Check sheet for the modelled part. Datum: model origin and axes. Units: mm. Coordinates: 2 decimals unless noted, no trailing zeros. Write each loop counter-clockwise with the first axis right and the second up, starting at its lowest first coordinate (ties: lowest second). Pieces come first, ordered by that corner, then holes. Notation, with made-up numbers: (-12.5, 61) -> (1.5, 61) arc R18 ccw to (1.5, 90) -> close; hole circle Ø5 at (-35.75, -21.5). An arc over 180 degrees is marked (long way). One line per item, written item: value. Start each with the question number.
1) Sectioned sample at C-C on x = -44.15. Enter the section's corners in (y, z), plus the area to 3 significant figures.
2) Sectioned sample at B-B on y = 3.75. Enter the section's corners in (x, z), plus the area to 3 significant figures.
3) Draft check along Z on faces 1 (the cylindrical face through (-6.5, 6.3, 0.1)), 2 (the flat face through (-29, 12.7, 0)), 3 (the flat face through (-28, 6, -25)), 4 (the flat face through (-29, 6, 25)). Enter one of: +Z half, -Z half, draft (parallel to the pull), parting line (faces both ways), or undercut.
4) Scan lines: line 1 along X through (y, z) = (8.25, 18.5); line 2 along Z through (x, y) = (-3.5, 2); line 3 along X through (y, z) = (5.75, 17). Record each from-to range of solid material in increasing order. Write a range as [from, to].
5) Gauge pin test, flat end, axial feed: P1, Ø3.5, axis at x = -44.15, z = 18.5, coming from the +Y side. Record the tip position at first contact, or that the pin passes through.
6) Sectioned sample at A-A on z = -18.5. Enter the section's corners in (x, y).
7) Sectioned sample at D-D on z = 0. Enter the section's corners in (x, y).
```python
from build123d import *

# Parameters (mm, degrees)
CROQUIS2_R              = 3
SALIENTE_EXTRUIR1_DEPTH = 12.7


with BuildPart() as part:
    # Croquis2 → Saliente-Extruir1 (new body)
    with BuildSketch(Plane(origin=(0, 0, 0), x_dir=(1, 0, 0), z_dir=(0, 1, 0))):
        with BuildLine():
            Line((0, 25), (-57.15, 25))
            Line((-57.15, 25), (-57.15, -25))
            Line((-57.15, -25), (0, -25))
            Line((0, -25), (0, -6.5))
            ThreePointArc((0, -6.5), (-6.5, 0), (0, 6.5))
            Line((0, 6.5), (0, 25))
        make_face()
        with Locations(Location((-44.15, -18.5, 0), (0, 0, 270))):
            Circle(CROQUIS2_R, mode=Mode.SUBTRACT)
        with Locations(Location((-44.15, 18.5, 0), (0, 0, 270))):
            Circle(CROQUIS2_R, mode=Mode.SUBTRACT)
    extrude(amount=SALIENTE_EXTRUIR1_DEPTH)


solid = part.part
```
Answers:
1. outline: (0, -25) -> (12.7, -25) -> (12.7, -21.5) -> (0, -21.5) -> close; (0, -15.5) -> (12.7, -15.5) -> (12.7, 15.5) -> (0, 15.5) -> close; (0, 21.5) -> (12.7, 21.5) -> (12.7, 25) -> (0, 25) -> close
1. area: 483 mm2
2. outline: (-57.15, -25) -> (0, -25) -> (0, -6.5) arc R6.5 cw to (0, 6.5) -> (0, 25) -> (-57.15, 25) -> close; hole circle Ø6 at (-44.15, -18.5); hole circle Ø6 at (-44.15, 18.5)
2. area: 2,730 mm2
3. face 1: undercut
3. face 2: draft
3. face 3: -Z half
3. face 4: +Z half
4. line 1: x = [-57.15, -47.15], [-41.15, 0]
4. line 2: z = [-25, -5.48], [5.48, 25]
4. line 3: x = [-57.15, -46.75], [-41.55, 0]
5. P1: passes through
6. outline: (-57.15, 0) -> (-47.15, 0) -> (-47.15, 12.7) -> (-57.15, 12.7) -> close; (-41.15, 0) -> (0, 0) -> (0, 12.7) -> (-41.15, 12.7) -> close
7. outline: (-57.15, 0) -> (-6.5, 0) -> (-6.5, 12.7) -> (-57.15, 12.7) -> close
